Autodesk Inventor part; units mm, degrees
ref_plane "YZ Plane" through (0, 0, 0) normal (1, 0, 0) x (0, 1, 0)
ref_plane "XZ Plane" through (0, 0, 0) normal (0, 1, 0) x (-1, 0, 0)
ref_plane "XY Plane" through (0, 0, 0) normal (0, 0, 1) x (1, 0, 0)
sketch "Sketch1" plane through (0, 0, 0) normal (0, 1, 0) x (-1, 0, 0)
  line L0 (-78.7139, 38.3135) -> (111.2861, 38.3135)
  line L1 (111.2861, 38.3135) -> (111.2861, -121.6865)
  line L2 (111.2861, -121.6865) -> (-78.7139, -121.6865)
  line L3 (-78.7139, -121.6865) -> (-78.7139, 38.3135)
  line L4 (111.2861, -6.6865) -> (116.2861, -6.6865)
  line L5 (116.2861, -6.6865) -> (116.2861, -36.6865)
  line L6 (116.2861, -36.6865) -> (111.2861, -36.6865)
  line L7 (111.2861, -36.6865) -> (111.2861, -6.6865)
  line L8 (111.2861, -66.6865) -> (116.2861, -66.6865)
  line L9 (116.2861, -66.6865) -> (116.2861, -96.6865)
  line L10 (116.2861, -96.6865) -> (111.2861, -96.6865)
  line L11 (111.2861, -96.6865) -> (111.2861, -66.6865)
  line L12 (111.2861, -41.6865) -> (-78.7139, -41.6865) construction
  line L13 (16.2861, 38.3135) -> (16.2861, -121.6865) construction
  line L14 (-78.7139, -6.6865) -> (-83.7139, -6.6865)
  line L15 (-83.7139, -6.6865) -> (-83.7139, -36.6865)
  line L16 (-83.7139, -36.6865) -> (-78.7139, -36.6865)
  line L17 (-78.7139, -66.6865) -> (-83.7139, -66.6865)
  line L18 (-83.7139, -66.6865) -> (-83.7139, -96.6865)
  line L19 (-83.7139, -96.6865) -> (-78.7139, -96.6865)
  line L20 (-78.7139, -41.6865) -> (111.2861, -41.6865) construction
  point P0 (0, 0)
  point P1 (-78.7139, -66.6865)
  point P2 (-78.7139, -96.6865)
  dimension "d0" = 190
  dimension "d1" = 160
  dimension "d2" = 5
  dimension "d3" = 30
  dimension "d4" = 5
  dimension "d5" = 30
  dimension "d6" = 30
  dimension "d7" = 5
extrude "Extrusion1" add sketch "Sketch1" along normal blind 5
properties part number "Tapa diagonal"
Geometry: final body of the model. Coordinates: model frame, mm. A direction names the side the tool comes from. Round coordinates to 2 decimals unless told otherwise and drop trailing zeros. Write each loop counter-clockwise with the first axis right and the second up, starting at its lowest first coordinate (ties: lowest second). Pieces come first, ordered by that corner, then holes. Notation, with made-up numbers: M -6.75,55 L 9.25,55 A21 cw 9.25,64 Z; hole C 17.5,22.5 d5. An arc over 180 degrees is marked long. Answer in a Markdown table with one row per item. Add a question column.
(1) Cut plane B-B, the plane z = -61. Return the cut outline in (x, y).
(2) Ray query, L1, parallel to X at y = 1.9, z = -112. Return the intervals inside material, ascending.
(3) Contact query for flat-ended pins moving along their axis: pin 1 (2.5 mm diameter, centred on x = -113.5, y = 3, fed in from -Z); pin 2 (1.5 mm diameter, centred on x = -112.5, y = 1.5, fed in from +Z); pin 3 (1.5 mm diameter, centred on y = 2.5, z = 10, fed in from -X). Output: stop coordinate, or through.
(4) Draft query along Z for faces 1 (the face through (-114, 2, -96.686)), 2 (the face through (-111.286, 2, -51)), 3 (the face through (78.714, 2, -52)), 4 (the face through (83.714, 2, -81)). Return one class per face: pulls with the +Z half, pulls with the -Z half, needs draft (parallel to the pull), parting line crosses it, or undercut.
(5) Reachability of faces 5 (the face through (-114, 2, -6.686)), 6 (the face through (78.714, 2, 15)), 7 (the face through (-114, 2, -66.686)), 8 (the face through (-111.286, 2, -109)), 9 (the face through (78.714, 2, -109)) from +Z, -Z, +X, -X, +Y, -Y: full face, straight path, thin tool, end or side. Return the list, or none.
(6) Cut plane A-A, the plane y = 0.9. Return the cut outline in (x, z), then the cut area to 3 significant figures.
Established:
| question | item | result |
|---|---|---|
| 1 | outline | M -111.29,0 L 78.71,0 L 78.71,5 L -111.29,5 Z |
| 2 | L1 | -111.29 to 78.71 |
| 3 | pin 1 | z = -96.69 |
| 3 | pin 2 | z = -6.69 |
| 3 | pin 3 | x = -111.29 |
| 4 | face 1 | pulls with the -Z half |
| 4 | face 2 | undercut |
| 4 | face 3 | undercut |
| 4 | face 4 | needs draft |
| 5 | face 5 | +Z, -X, +Y, -Y |
| 5 | face 6 | +Z, +X, +Y, -Y |
| 5 | face 7 | -X, +Y, -Y |
| 5 | face 8 | -Z, -X, +Y, -Y |
| 5 | face 9 | -Z, +X, +Y, -Y |
| 6 | outline | M -116.29,-96.69 L -111.29,-96.69 L -111.29,-121.69 L 78.71,-121.69 L 78.71,-96.69 L 83.71,-96.69 L 83.71,-66.69 L 78.71,-66.69 L 78.71,-36.69 L 83.71,-36.69 L 83.71,-6.69 L 78.71,-6.69 L 78.71,38.31 L -111.29,38.31 L -111.29,-6.69 L -116.29,-6.69 L -116.29,-36.69 L -111.29,-36.69 L -111.29,-66.69 L -116.29,-66.69 Z |
| 6 | area | 31,000 mm² |
